Check sheet for the modelled part. Datum: model origin and axes. Units: mm. Round coordinates to 2 decimals unless told otherwise and drop trailing zeros. Write each loop counter-clockwise with the first axis right and the second up, starting at its lowest first coordinate (ties: lowest second). Pieces come first, ordered by that corner, then holes.
Item 1: Material ranges on line 1 along Z through (x, y) = (9, -18.5); line 2 along Z through (x, y) = (0, -6.5); line 3 along Y through (x, z) = (-6, -53.5), recorded low to high.
Item 2: Section check A-A, the plane y = -24.5. Record the cut outline in (x, z), plus the area to 3 significant figures.
Item 3: Section check B-B, the plane y = -31.5. Record the cut outline in (x, z), plus the area to 3 significant figures.
Item 4: Depth check by flat-ended pin: pin 1 (6 mm diameter, centred on y = -7, z = -39, fed in from -X); pin 2 (2 mm diameter, centred on x = -29, z = -42, fed in from -Y); pin 3 (1 mm diameter, centred on y = -31, z = 28, fed in from +X); pin 4 (2 mm diameter, centred on x = -44, z = 44, fed in from +Y). Enter the tip coordinate at first touch or a pass-through.
from build123d import *

# Parameters (mm, degrees)
FILLET2_R = 5
FILLET3_R = 5
FILLET4_R = 6


with BuildPart() as part:
    # Sketch1 → Revolve3 (revolve)
    with BuildSketch(Plane.XY, mode=Mode.PRIVATE) as revolve3_sk:
        Polygon((0, -44.99102057), (25, -44.99102057), (60, -19.99102057), (60, 5.00897943), (0, 5.00897943), align=None)
    revolve(revolve3_sk.sketch.rotate(Axis((0, 5.00897943, 0), (0, -1, 0)), 180), axis=Axis((0, 5.00897943, 0), (0, -1, 0)))

    # Fillet2
    fillet2_edges = [part.edges().sort_by_distance(p)[0] for p in [
        (60, 5.00897943, 0),
    ]]
    fillet(fillet2_edges, radius=FILLET2_R)

    # Fillet3
    fillet3_edges = [part.edges().sort_by_distance(p)[0] for p in [
        (60, -19.99102057, 0),
    ]]
    fillet(fillet3_edges, radius=FILLET3_R)

    # Fillet4
    fillet4_edges = [part.edges().sort_by_distance(p)[0] for p in [
        (25, -44.99102057, 0),
    ]]
    fillet(fillet4_edges, radius=FILLET4_R)


solid = part.part
Values found:
1. line 1: z = -59.2 to 59.2
1. line 2: z = -60 to 60
1. line 3: y = -24.39 to 5.01
2. outline: circle Ø107.37 at (0, 0)
2. area: 9,060 mm2
3. outline: circle Ø87.77 at (0, 0)
3. area: 6,050 mm2
4. pin 1: stops at x = -48
4. pin 2: stops at y = -27.11
4. pin 3: stops at x = 35.68
4. pin 4: passes through
